Geometry: see drawing. Coordinates: mm, zero at the bounding-box minimum. Coordinates: 2 decimals unless noted, no trailing zeros. Loops run counter-clockwise (first coordinate to the right, second up) from the corner with the lowest first, then second, coordinate; pieces in that order, holes last.
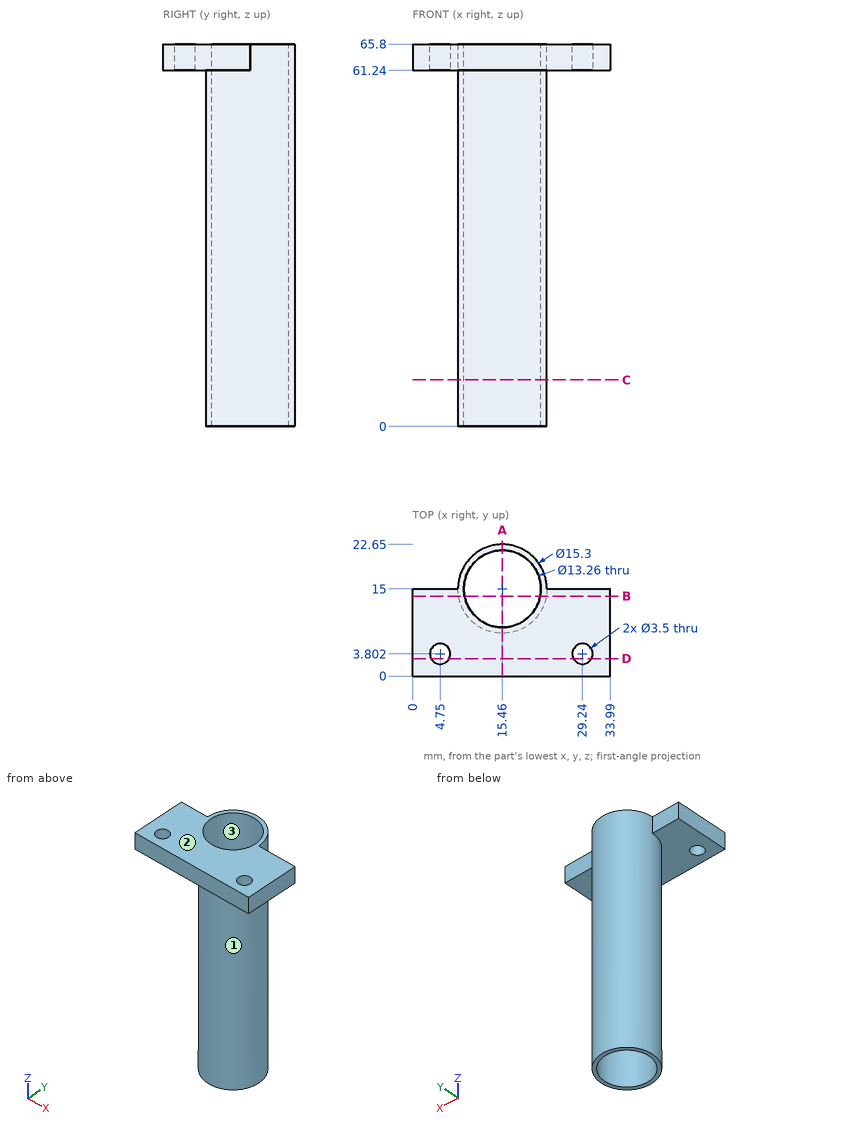
Item 1: Section query C-C (z = 8). Output: boundary loops of the cut face in (x, y), then the cut area to 3 significant figures.
Result:
outline: circle Ø15.3 at (15.46, 15); hole circle Ø13.26 at (15.46, 15)
area: 45.8 mm2
Item 2: Line query: L1, parallel to X at y = 15, z = 40; L2, parallel to Y at x = 15, z = 56; L3, parallel to Y at x = 4.75, z = 64.3. Output: solid intervals per line, ascending.
Result:
L1: x = 7.81 to 8.83, 22.09 to 23.11
L2: y = 7.36 to 8.39, 21.61 to 22.64
L3: y = 0 to 2.05, 5.55 to 15
Item 3: Section query A-A (x = 15.46). Output: boundary loops of the cut face in (y, z).
Result:
outline: (0, 61.24) - (7.35, 61.24) - (7.35, 0) - (8.37, 0) - (8.37, 65.8) - (0, 65.8) - close; (21.63, 0) - (22.65, 0) - (22.65, 65.8) - (21.63, 65.8) - close
Item 4: Section query D-D (y = 3). Output: boundary loops of the cut face in (x, z).
Result:
outline: (0, 61.24) - (3.19, 61.24) - (3.19, 65.8) - (0, 65.8) - close; (6.31, 61.24) - (27.68, 61.24) - (27.68, 65.8) - (6.31, 65.8) - close; (30.8, 61.24) - (33.99, 61.24) - (33.99, 65.8) - (30.8, 65.8) - close
Item 5: Contact query for flat-ended pins moving along their axis: P1, Ø1.4, axis at x = 29, z = 63.5, coming from the +Y side; P2, Ø1.5, axis at y = 15, z = 15.5, coming from the +X side; P3, Ø4, axis at y = 6, z = 14.5, coming from the -X side. Output: stop coordinate, or through.
Result:
P1: stops at y = 15
P2: stops at x = 23.11
P3: stops at x = 12.37
Item 6: Section query B-B (y = 13.75). Output: boundary loops of the cut face in (x, z).
Result:
outline: (0, 61.24) - (7.91, 61.24) - (7.91, 0) - (8.95, 0) - (8.95, 65.8) - (0, 65.8) - close; (21.97, 0) - (23.01, 0) - (23.01, 61.24) - (33.99, 61.24) - (33.99, 65.8) - (21.97, 65.8) - close
Item 7: Mould query, pull axis Y, two halves, no side actions, for the marked faces 1, 2 and 3. Classes: +Y half, -Y half, draft (parallel to the pull), parting line (faces both ways), or undercut.
Result:
face 1: parting line
face 2: draft
face 3: undercut
